For this review, take the finished solid that the model builds, in its own axes (mm). A direction names the side the tool comes from. Round coordinates to 2 decimals unless told otherwise and drop trailing zeros. Loops run counter-clockwise (first coordinate to the right, second up) from the corner with the lowest first, then second, coordinate; pieces in that order, holes last.
1) Take a section at B-B (z = 0). State the section outline as (x, y) points, then the cut area to 3 significant figures.
2) Take a section at C-C (y = -6). State the section outline as (x, z) points, then the cut area to 3 significant figures.
3) Take a section at D-D (x = -41). State the section outline as (y, z) points, then the cut area to 3 significant figures.
4) Insertion check: pin 1 (3 mm diameter, centred on y = -30, z = 7.5, fed in from -X); pin 2 (10 mm diameter, centred on y = -4, z = -6, fed in from -X); pin 3 (10 mm diameter, centred on y = -5, z = 8.5, fed in from -X). Each pin has a flat end and moves straight along its axis. Give the tip position at first contact, or say it passes through.
5) Mouldability with a two-part tool opening along Z and no side actions: class faces 6 (the cylindrical face through (-45.67, -12.32, 0.34)), 7 (the cylindrical face through (-25.74, -12.59, 12.95)), 8 (the flat face through (-38, 0.5, 0)) as pulls with the +Z half, pulls with the -Z half, needs draft (parallel to the pull), parting line crosses it, or undercut.
6) Tool access review of faces 1 (the cylindrical face through (-25.74, -12.59, -17.05)), 2 (the cylindrical face through (-24.4, -0.07, -0.19)), 3 (the cylindrical face through (-30.81, -12.606, 12.602)), 4 (the flat face through (-35, -29, 0)), 5 (the flat face through (-25, -31.5, 0)): name each direction out of +Z, -Z, +X, -X, +Y, -Y from which nothing blocks a thin tool from reaching the whole face with its end or side.
7) Wall thickness on L1, parallel to Z at x = -26.2, y = -12.5; L2, parallel to Y at x = -32, z = -15; L3, parallel to Z at x = -35, y = -23: over which ranges is each line inside the solid? List them lowest first.
8) Take a section at A-A (x = -17). State the section outline as (y, z) points, then the cut area to 3 significant figures.
```python
from build123d import *

# Parameters (mm, degrees)
PAD001_DEPTH    = 26
SKETCH003_R     = 2.05
POCKET_DEPTH    = 12
SKETCH005_R     = 2.4
POCKET001_DEPTH = 10.5
PAD004_DEPTH    = 10
FILLET006_R     = 2
FILLET007_R     = 0.5
FILLET008_R     = 2


with BuildPart() as part:
    # Sketch001 → Pad001 (new body)
    with BuildSketch(Plane.XZ):
        with BuildLine():
            ThreePointArc((-35, 21), (-45.67029, 0), (-35, -21))
            Line((-35, -21), (-25, -28.299822))
            Line((-25, 28.299822), (-25, -28.299822))
            Line((-35, 21), (-25, 28.299822))
        make_face()
    extrude(amount=PAD001_DEPTH)

    # Sketch003 (on Face3 of Pad001) → Pocket (cut)
    with BuildSketch(Plane(origin=(-25, 0, 0), x_dir=(0, 0, 1), z_dir=(1, 0, 0))):
        with Locations((-15, 13)):
            Circle(SKETCH003_R)
        with Locations((15, 13)):
            Circle(SKETCH003_R)
    extrude(amount=-POCKET_DEPTH, mode=Mode.SUBTRACT)

    # Sketch005 (on Face9 of Pocket) → Pocket001 (cut)
    with BuildSketch(Plane(origin=(-37, 0, 0), x_dir=(0, 0, 1), z_dir=(1, 0, 0))):
        with Locations((-15, 13)):
            Circle(SKETCH005_R)
        with Locations((15, 13)):
            Circle(SKETCH005_R)
    extrude(amount=POCKET001_DEPTH, mode=Mode.SUBTRACT)

    # Sketch006 (on Face6 of Pocket001) → Pad004 (join, symmetric)
    with BuildSketch(Plane(origin=(-25, 0, 0), x_dir=(0, 0, 1), z_dir=(1, 0, 0))):
        Polygon((-13.504032, 26), (13.504032, 26), (15, 32), (-15, 32), align=None)
        Polygon((-13.504032, 0), (13.504032, 0), (15, -6), (-15, -6), align=None)
    extrude(amount=PAD004_DEPTH, both=True)

    # Fillet006
    fillet006_edges = [part.edges().sort_by_distance(p)[0] for p in [
        (-25, -26, 0),
        (-25, 0, 0),
        (-35, 0, 0),
        (-35, -26, 0),
    ]]
    fillet(fillet006_edges, radius=FILLET006_R)

    # Fillet007
    fillet007_edges = [part.edges().sort_by_distance(p)[0] for p in [
        (-15, 6, 0),
        (-25, 6, -15),
        (-35, 6, 0),
        (-25, 6, 15),
        (-25, -32, 15),
        (-15, -32, 0),
        (-25, -32, -15),
        (-35, -32, 0),
    ]]
    fillet(fillet007_edges, radius=FILLET007_R)

    # Fillet008
    fillet008_edges = [part.edges().sort_by_distance(p)[0] for p in [
        (-37, -13, 12.6),
        (-37, -13, -17.4),
    ]]
    fillet(fillet008_edges, radius=FILLET008_R)


with BuildPart() as part_1:
    # Body001 placement: moved
    add(part.part.moved(Location((0, 0.5, 0))))


solid = part_1.part
```
Response:
1. outline: (-45.67, -25.5) - (-37, -25.5) arc R2 cw to (-35, -27.5) - (-35, -31) arc R0.5 ccw to (-34.5, -31.5) - (-15.5, -31.5) arc R0.5 ccw to (-15, -31) - (-15, -25.5) - (-23, -25.5) arc R2 cw to (-25, -23.5) - (-25, -1.5) arc R2 cw to (-23, 0.5) - (-15, 0.5) - (-15, 6) arc R0.5 ccw to (-15.5, 6.5) - (-34.5, 6.5) arc R0.5 ccw to (-35, 6) - (-35, 2.5) arc R2 cw to (-37, 0.5) - (-45.67, 0.5) - close
1. area: 781 mm2
2. outline: (-35, -21) - (-25, -28.3) - (-25, 28.3) - (-35, 21) arc R26 ccw to start
2. area: 807 mm2
3. outline: (-25.5, -14.87) - (0.5, -14.87) - (0.5, 14.87) - (-25.5, 14.87) - close
3. area: 773 mm2
4. pin 1: stops at x = -35
4. pin 2: stops at x = -45.65
4. pin 3: stops at x = -45.43
5. face 6: parting line crosses it
5. face 7: undercut
5. face 8: needs draft
6. face 1: +X
6. face 2: +Z, -Z, +X
6. face 3: none
6. face 4: +Z, -Z, -X, -Y
6. face 5: +Z, -Z, +X, -X, -Y
7. L1: z = -27.42 to -17.05, -12.95 to 12.95, 17.05 to 27.42
7. L2: y = -25.5 to -14.9, -10.1 to 0.5
7. L3: z = -21 to 21
8. outline: (-31.5, -14.36) arc R0.5 ccw to (-30.88, -14.85) - (-25.5, -13.5) - (-25.5, 13.5) - (-30.88, 14.85) arc R0.5 ccw to (-31.5, 14.36) - close; (0.5, -13.5) - (5.88, -14.85) arc R0.5 ccw to (6.5, -14.36) - (6.5, 14.36) arc R0.5 ccw to (5.88, 14.85) - (0.5, 13.5) - close
8. area: 342 mm2
